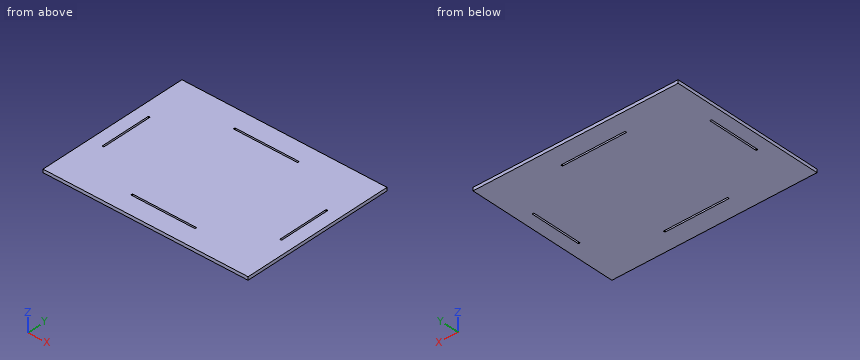
from build123d import *

# Parameters (mm, degrees)
F0_W     = 406.4
F0_H     = 304.8
F0_W_2   = 127
F0_H_2   = 3.4163
F0_W_3   = 3.4163
F0_H_3   = 101.6
F1_DEPTH = 6.35


with BuildPart() as f1:
    # F0 (on Top) → F1 (new body)
    with BuildSketch(Plane.XY):
        Rectangle(F0_W, F0_H)
        with Locations((0, -112.59185)):
            Rectangle(F0_W_2, F0_H_2, mode=Mode.SUBTRACT)
        with Locations((-176.09185, 0)):
            Rectangle(F0_W_3, F0_H_3, mode=Mode.SUBTRACT)
        with Locations((0, 112.59185)):
            Rectangle(F0_W_2, F0_H_2, mode=Mode.SUBTRACT)
        with Locations((176.09185, 0)):
            Rectangle(F0_W_3, F0_H_3, mode=Mode.SUBTRACT)
    extrude(amount=-F1_DEPTH)


solid = f1.part
Can you work these out from the model? Positions are in its coordinate system, mm. Round coordinates to 2 decimals unless told otherwise and drop trailing zeros. Loops run counter-clockwise (first coordinate to the right, second up) from the corner with the lowest first, then second, coordinate; pieces in that order, holes last. Notation, with made-up numbers: (34, 78.5) - (39, 78.5) arc R13 ccw to (39, 102.5) - close; hole circle Ø4 at (57.25, 40). An arc over 180 degrees is marked (long way). Answer in a Markdown table with one row per item. Add a question column.
Q1. I want a section at B-B on y = 25. List the corners of the cut face in (x, z) for me, and give its area (3 significant figures).
Q2. I want a section at A-A on x = -29. List the corners of the cut face in (y, z) for me.
Q3. I need wall thicknesses on L1, parallel to X at y = 46, z = -4.5; L2, parallel to Y at x = 12, z = -2.5. Which ranges of each line are inside material? Lowest first, please.
A:
| question | item | result |
|---|---|---|
| 1 | outline | (-203.2, -6.35) - (-177.8, -6.35) - (-177.8, 0) - (-203.2, 0) - close; (-174.38, -6.35) - (174.38, -6.35) - (174.38, 0) - (-174.38, 0) - close; (177.8, -6.35) - (203.2, -6.35) - (203.2, 0) - (177.8, 0) - close |
| 1 | area | 2,540 mm^2 |
| 2 | outline | (-152.4, -6.35) - (-114.3, -6.35) - (-114.3, 0) - (-152.4, 0) - close; (-110.88, -6.35) - (110.88, -6.35) - (110.88, 0) - (-110.88, 0) - close; (114.3, -6.35) - (152.4, -6.35) - (152.4, 0) - (114.3, 0) - close |
| 3 | L1 | -203.2 to -177.8, -174.38 to 174.38, 177.8 to 203.2 |
| 3 | L2 | -152.4 to -114.3, -110.88 to 110.88, 114.3 to 152.4 |
